Read the model definition and answer for the solid it produces. Units are mm, in the model's axes. Face numbers are marked on the shaded views. A direction names the side the tool comes from. Coordinates: 2 decimals unless noted, no trailing zeros. Order: outer loops, then holes, each group sorted by start corner. A loop starts at its lowest first (then second) coordinate and runs counter-clockwise, first axis right, second up. Notation, with made-up numbers: M 43,28.25 L 67,28.25 A29 cw 67,55.25 Z; hole C 21.5,-9.75 d9. An arc over 180 degrees is marked long. One line per question, with ' | ' between items. Start each with the question number.
1) A tool of negligible diameter and unlimited length cuts with its end or side. For the marked faces 1, 2, 3, 4 and 5, from which of +Z, -Z, +X, -X, +Y, -Y can it reach the whole face along a straight path? Write none if from no direction.
2) Consider probe 1 along Y at (x, z) = (19.5, 12.1); probe 2 along Z at (x, y) = (28.5, -5); probe 3 along Z at (x, y) = (21.25, -0.5). Determine where each line is inside the solid, lowest interval first.
3) Find section C-C, the plane z = 12.6. Write down the section's boundary in (x, y).
4) Find section D-D, the plane y = 11.75. Write down the section's boundary in (x, z).
5) Find section A-A, the plane y = 4.5. Write down the section's boundary in (x, z), plus the area to 3 significant figures.
6) Given P1, Ø2, axis at y = 1, z = 11.5, coming from the +X side; P2, Ø1.2, axis at y = 3.5, z = 12, coming from the -X side; P3, Ø2, axis at x = 22.5, z = 11.5, coming from the +Y side, each flat-ended and moving along its own axis, determine where each tip first touches the part or whether it passes through.
7) Find section B-B, the plane x = 21.5. Write down the section's boundary in (y, z), plus the area to 3 significant figures.
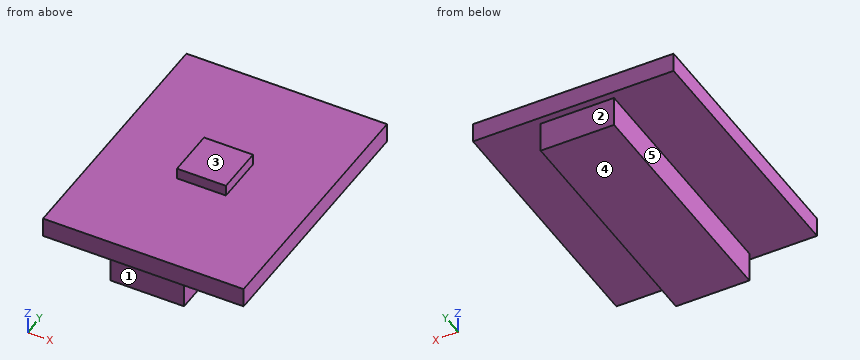
from build123d import *

# Parameters (mm, degrees)
SKETCH1_W           = 16.4
SKETCH1_H           = 21.2
BOSS_EXTRUDE1_DEPTH = 1.6
SKETCH2_W           = 6
SKETCH2_H           = 20
BOSS_EXTRUDE2_DEPTH = 2.5
SKETCH3_W           = 4
SKETCH3_H           = 4
BOSS_EXTRUDE3_DEPTH = 0.9


with BuildPart() as part:
    # Sketch1 → Boss-Extrude1 (new body)
    with BuildSketch(Plane.XY.offset(13.1)):
        with Locations((22, 3)):
            Rectangle(SKETCH1_W, SKETCH1_H)
    extrude(amount=BOSS_EXTRUDE1_DEPTH)

    # Sketch2 → Boss-Extrude2 (add)
    with BuildSketch(Plane.XY.offset(10.6)):
        with Locations((22, 3)):
            Rectangle(SKETCH2_W, SKETCH2_H)
    extrude(amount=BOSS_EXTRUDE2_DEPTH)

    # Sketch3 → Boss-Extrude3 (add)
    with BuildSketch(Plane.XY.offset(14.7)):
        with Locations((22, 3)):
            Rectangle(SKETCH3_W, SKETCH3_H)
    extrude(amount=BOSS_EXTRUDE3_DEPTH)


solid = part.part
Report:
1) face 1: -Z, +X, -X, -Y | face 2: -Z, +X, -X, +Y | face 3: +Z, +X, -X, +Y, -Y | face 4: -Z, +X, -X, +Y, -Y | face 5: -Z, -X, +Y, -Y
2) probe 1: y = -7 to 13 | probe 2: z = 13.1 to 14.7 | probe 3: z = 10.6 to 14.7
3) outline: M 19,-7 L 25,-7 L 25,13 L 19,13 Z
4) outline: M 13.8,13.1 L 19,13.1 L 19,10.6 L 25,10.6 L 25,13.1 L 30.2,13.1 L 30.2,14.7 L 13.8,14.7 Z
5) outline: M 13.8,13.1 L 19,13.1 L 19,10.6 L 25,10.6 L 25,13.1 L 30.2,13.1 L 30.2,14.7 L 24,14.7 L 24,15.6 L 20,15.6 L 20,14.7 L 13.8,14.7 Z | area: 44.8 mm^2
6) P1: stops at x = 25 | P2: stops at x = 19 | P3: stops at y = 13
7) outline: M -7.6,13.1 L -7,13.1 L -7,10.6 L 13,10.6 L 13,13.1 L 13.6,13.1 L 13.6,14.7 L 5,14.7 L 5,15.6 L 1,15.6 L 1,14.7 L -7.6,14.7 Z | area: 87.5 mm^2
